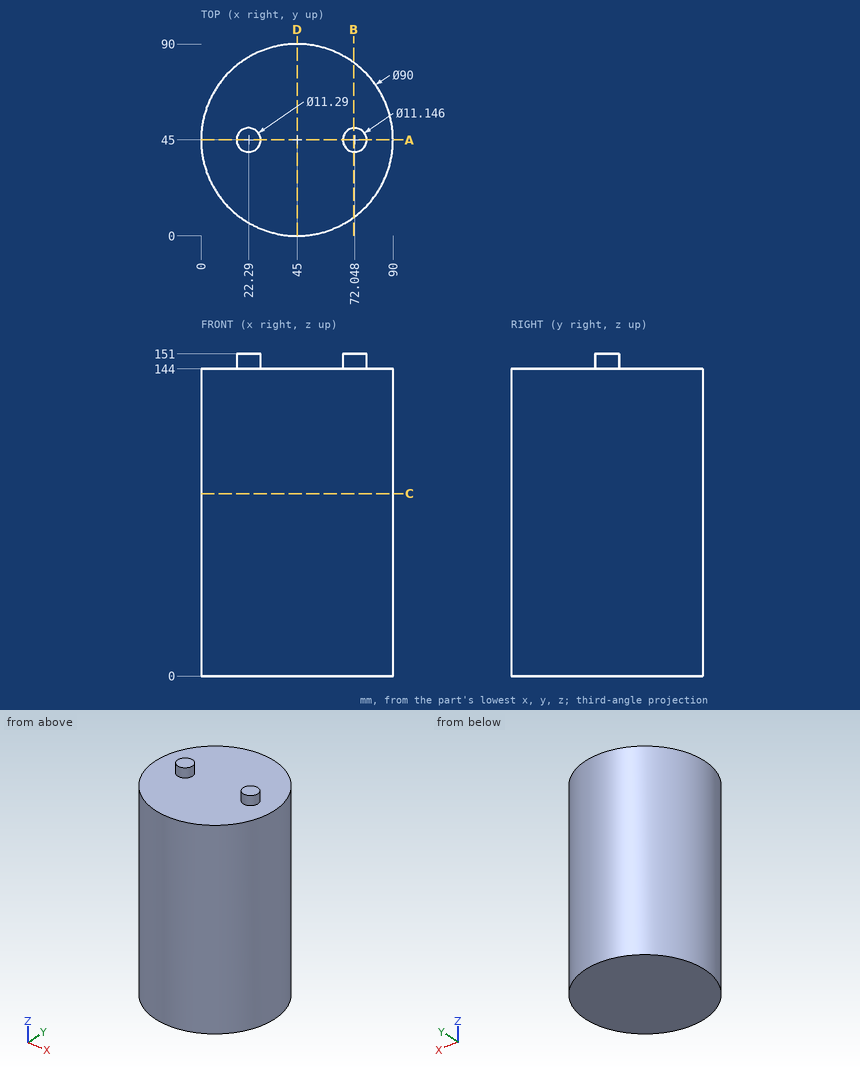
Job drawing, mm, ordinate dimensions from the low corner. One solid piece. Give positions to 0.01 mm unless a question says otherwise; leave off trailing zeros. Loops run counter-clockwise (first coordinate to the right, second up) from the corner with the lowest first, then second, coordinate; pieces in that order, holes last. Notation, with made-up numbers: M 49.5,-9.75 L 100.5,-9.75 A28 ccw 100.5,11.25 Z; hole C 69,57 d7. An arc over 180 degrees is marked long. Return JSON: item names as keys, results as strings.
1) Saw through at A-A, the plane y = 45. List the corners of the cut face in (x, z) (1 decimal).
Calculated:
{"outline": "M 0,0 L 90,0 L 90,144 L 77.6,144 L 77.6,151 L 66.5,151 L 66.5,144 L 27.9,144 L 27.9,151 L 16.6,151 L 16.6,144 L 0,144 Z"}
2) Saw through at B-B, the plane x = 71.5. List the corners of the cut face in (y, z).
Calculated:
{"outline": "M 8.63,0 L 81.37,0 L 81.37,144 L 50.55,144 L 50.55,151 L 39.45,151 L 39.45,144 L 8.63,144 Z"}
3) Drill centre lines: line 1 (Z direction, x = 58.5, y = 85); line 2 (Y direction, x = 49, z = 32.5); line 3 (Y direction, x = 54, z = 90). Where is each one in solid material? Low to high.
Calculated:
{"line 1": "z = 0 to 144", "line 2": "y = 0.18 to 89.82", "line 3": "y = 0.91 to 89.09"}
4) Saw through at D-D, the plane x = 45. List the corners of the cut face in (y, z), then the cut area to 3 significant figures.
Calculated:
{"outline": "M 0,0 L 90,0 L 90,144 L 0,144 Z", "area": "13,000 mm2"}
5) Flat gauge pins, fed straight in: pin 1 Ø5 at (x, y) = (12, 79) entering from +Z; pin 2 Ø10 at (x, z) = (27, 93.5) entering from +Y; pin 3 Ø3 at (x, z) = (46, 86) entering from +Y. Where does each tip first touch, or does it go through?
Calculated:
{"pin 1": "stops at z = 144", "pin 2": "stops at y = 88.08", "pin 3": "stops at y = 90"}
6) Saw through at C-C, the plane z = 85.5. List the corners of the cut face in (x, y), then the cut area to 3 significant figures.
Calculated:
{"outline": "C 45,45 d90", "area": "6,360 mm2"}
